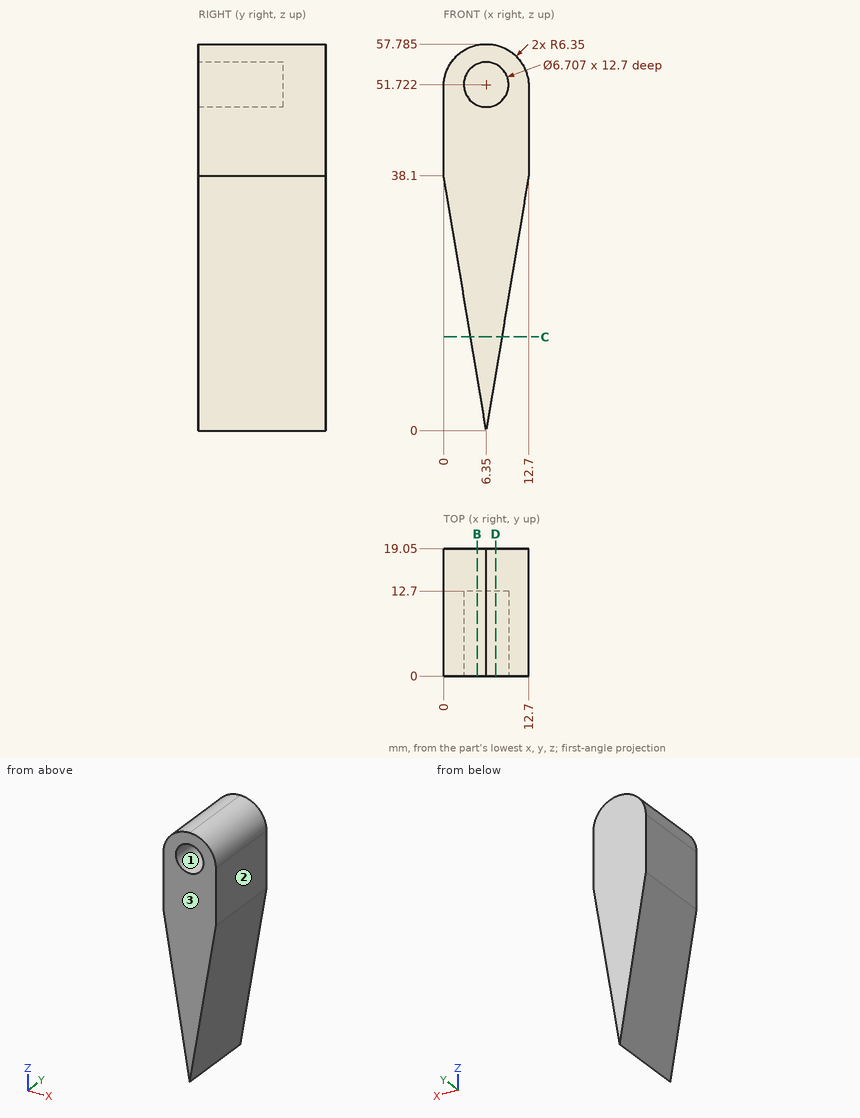
Job drawing, mm, ordinate dimensions from the low corner. One solid piece. Round coordinates to 2 decimals unless told otherwise and drop trailing zeros. Loops run counter-clockwise (first coordinate to the right, second up) from the corner with the lowest first, then second, coordinate; pieces in that order, holes last.
Item 1: Cut at C-C, the plane z = 14. Give the cut face in (x, y), then the cut area to 3 significant figures.
Item 2: Cut at B-B, the plane x = 5. Give the cut face in (y, z), then the cut area to 3 significant figures.
Item 3: Mould opens along X. For the marked faces 1, 2 and 3 say: +X half, -X half, draft (parallel to the pull), parting line (faces both ways), or undercut.
Item 4: Drill centre lines: line 1 (X direction, y = 5, z = 3.5); line 2 (X direction, y = 1, z = 4). Where is each one in solid material? Low to high.
Item 5: Drop flat-ended pins along their axis: P1, Ø6, axis at y = 14.5, z = 8, coming from the -X side; P2, Ø5, axis at y = 16, z = 20.5, coming from the -X side; P3, Ø8, axis at y = 2.5, z = 25.5, coming from the -X side. Give the stop position or say it passes through.
Item 6: Cut at D-D, the plane x = 7.75. Give the cut face in (y, z).
A:
1. outline: (4.02, 0) - (8.68, 0) - (8.68, 19.05) - (4.02, 19.05) - close
1. area: 88.9 mm2
2. outline: (0, 8.1) - (19.05, 8.1) - (19.05, 57.64) - (0, 57.64) - (0, 54.79) - (12.7, 54.79) - (12.7, 48.65) - (0, 48.65) - close
2. area: 866 mm2
3. face 1: undercut
3. face 2: +X half
3. face 3: draft
4. line 1: x = 5.77 to 6.93
4. line 2: x = 5.68 to 7.02
5. P1: stops at x = 4.52
5. P2: stops at x = 2.52
5. P3: stops at x = 1.43
6. outline: (0, 8.4) - (19.05, 8.4) - (19.05, 57.63) - (0, 57.63) - (0, 54.77) - (12.7, 54.77) - (12.7, 48.67) - (0, 48.67) - close
